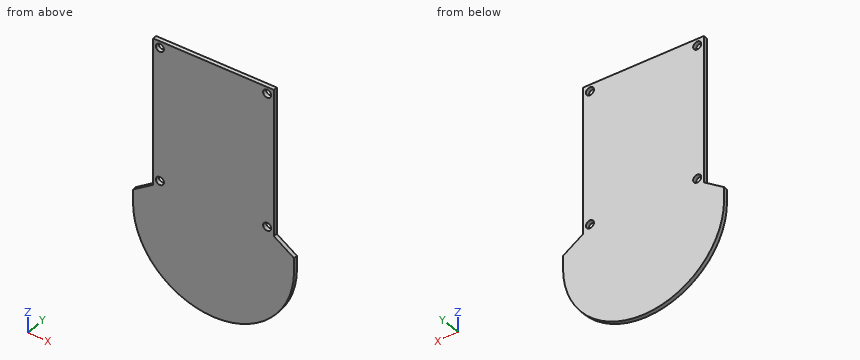
from build123d import *

# Parameters (mm, degrees)
BOSS_EXTRUDE1_DEPTH = 1.5
SKETCH2_R           = 1.5
CUT_EXTRUDE1_DEPTH  = 2.5


with BuildPart() as part:
    # Sketch1 → Boss-Extrude1 (new body)
    with BuildSketch(Plane(origin=(0, 0, 0), x_dir=(1, 0, 0), z_dir=(0, 1, 0))):
        with BuildLine():
            Line((-45.021006533, 42.5), (-45.021006533, 37.5))
            Line((-45.021006533, 37.5), (-37.5, 32.5))
            Line((-37.5, 32.5), (-37.5, -22.5))
            Line((-37.5, -22.5), (7.5, -22.5))
            Line((7.5, -22.5), (7.5, 32.5))
            Line((7.5, 32.5), (15.021006533, 37.5))
            Line((15.021006533, 37.5), (15.021006533, 42.5))
            ThreePointArc((15.021006533, 42.5), (-15, 72.521006533), (-45.021006533, 42.5))
        make_face()
    extrude(amount=BOSS_EXTRUDE1_DEPTH)

    # Sketch2 → Cut-Extrude1 (cut, through all)
    with BuildSketch(Plane(origin=(0, 1.5, 0), x_dir=(1, 0, 0), z_dir=(0, 1, 0))):
        with Locations((-35, 30)):
            Circle(SKETCH2_R)
        with Locations((-35, -20)):
            Circle(SKETCH2_R)
        with Locations((5, -20)):
            Circle(SKETCH2_R)
        with Locations((5, 30)):
            Circle(SKETCH2_R)
    extrude(amount=-CUT_EXTRUDE1_DEPTH, mode=Mode.SUBTRACT)


solid = part.part
Here's how the part is built. I have some questions about the finished solid (model axes, mm). Give positions to 0.01 mm unless a question says otherwise; leave off trailing zeros. Loops run counter-clockwise (first coordinate to the right, second up) from the corner with the lowest first, then second, coordinate; pieces in that order, holes last. Notation, with made-up numbers: (49, 69) -> (101, 69) arc R24 cw to (101, 102) -> close; hole circle Ø5 at (28, 9). An arc over 180 degrees is marked (long way). One line per item, written item: value.
Q1. I'm going to push flat-ended pins straight in: pin 1 Ø2.5 at (x, z) = (-35, -30) entering from +Y; pin 2 Ø0.8 at (y, z) = (0.5, -2) entering from +X; pin 3 Ø5 at (x, z) = (5, 20) entering from +Y. Where does each tip first touch, or does it pass through?
Answers follow:
pin 1: through
pin 2: x = 7.5
pin 3: y = 1.5
Q2. Suppose I cut it at D-D on x = -30. Please give me the cut outline in (y, z), then the cut area to 3 significant figures.
Answers follow:
outline: (0, -68.51) -> (1.5, -68.51) -> (1.5, 22.5) -> (0, 22.5) -> close
area: 137 mm^2
Q3. Suppose I cut it at A-A on z = -30. Please give me the cut outline in (x, y).
Answers follow:
outline: (-37.5, 0) -> (-36.5, 0) -> (-36.5, 1.5) -> (-37.5, 1.5) -> close; (-33.5, 0) -> (3.5, 0) -> (3.5, 1.5) -> (-33.5, 1.5) -> close; (6.5, 0) -> (7.5, 0) -> (7.5, 1.5) -> (6.5, 1.5) -> close
Q4. If I drill on line 1 along X through (y, z) = (0.6, -30); line 2 along Z through (x, y) = (5, 0.8); line 3 along X through (y, z) = (0.2, -3.5), over which ranges is the centre line in solid material (lowest first)?
Answers follow:
line 1: -37.5 to -36.5, -33.5 to 3.5, 6.5 to 7.5
line 2: -64.89 to -31.5, -28.5 to 18.5, 21.5 to 22.5
line 3: -37.5 to 7.5
Q5. Suppose I cut it at B-B on y = 1.2. Please give me the cut outline in (x, z), then the cut area to 3 significant figures.
Answers follow:
outline: (-45.02, -42.5) arc R30.02 ccw to (15.02, -42.5) -> (15.02, -37.5) -> (7.5, -32.5) -> (7.5, 22.5) -> (-37.5, 22.5) -> (-37.5, -32.5) -> (-45.02, -37.5) -> close; hole circle Ø3 at (-35, -30); hole circle Ø3 at (-35, 20); hole circle Ø3 at (5, -30); hole circle Ø3 at (5, 20)
area: 4,430 mm^2
Q6. Suppose I cut it at C-C on x = 5. Please give me the cut outline in (y, z), then the cut area to 3 significant figures.
Answers follow:
outline: (0, -64.89) -> (1.5, -64.89) -> (1.5, -31.5) -> (0, -31.5) -> close; (0, -28.5) -> (1.5, -28.5) -> (1.5, 18.5) -> (0, 18.5) -> close; (0, 21.5) -> (1.5, 21.5) -> (1.5, 22.5) -> (0, 22.5) -> close
area: 122 mm^2
